Autodesk Inventor part; units mm, degrees
ref_plane "YZ Plane" through (0, 0, 0) normal (1, 0, 0) x (0, 1, 0)
ref_plane "XZ Plane" through (0, 0, 0) normal (0, 1, 0) x (-1, 0, 0)
ref_plane "XY Plane" through (0, 0, 0) normal (0, 0, 1) x (1, 0, 0)
sketch "Sketch1" plane through (0, 0, 0) normal (1, 0, 0) x (0, 1, 0)
  line L0 (0, 0) -> (25.4, 0)
  line L1 (25.4, 0) -> (25.4, -50.8)
  line L2 (25.4, -50.8) -> (0, -50.8)
  line L3 (0, -50.8) -> (0, 0)
  circle A0 centre (12.7, -12.9077) radius 2.75
  circle A1 centre (12.7, -40.4254) radius 2.75
  dimension "d0" = 25.4
  dimension "d1" = 50.8
  dimension "d2" = 5.5
  dimension "d3" = 5.5
extrude "Extrusion1" add sketch "Sketch1" along normal blind 10
sketch "Sketch2" plane through (0, 0, 0) normal (-1, 0, 0) x (0, 0, 1)
  line L0 (-50.8, 0) -> (-50.8, 25.4)
  line L1 (0, 0) -> (-50.8, 0)
  line L2 (0, 25.4) -> (0, 0)
  line L3 (-50.8, 25.4) -> (0, 25.4)
  circle A0 centre (-40.4254, 12.7) radius 2.75
  circle A1 centre (-12.9077, 12.7) radius 2.75
  line L4 (2.3448, 23.6998) -> (5.142, 21.6715)
  line L5 (3.7285, 30.542) -> (1.7002, 27.7448)
  line L6 (20.0524, 42.2345) -> (17.2552, 44.2628)
  line L7 (22.2632, 12.8343) -> (24.2915, 15.6316)
  line L8 (15.4211, 14.2181) -> (18.2183, 12.1898)
  line L9 (0, 25.4) -> (14.9104, 45.963)
  line L10 (14.9104, 45.963) -> (6.8148, 51.8333)
  line L11 (-12.3523, 25.4) -> (6.8148, 51.8333)
  line L12 (0, 25.4) -> (20.563, 10.4896)
  line L13 (20.563, 10.4896) -> (0, 0)
  line L14 (-50.8, 25.4) -> (0, 25.4)
  line L15 (0, 25.4) -> (0, 35.4)
  line L16 (0, 35.4) -> (-50.8, 35.4)
  line L17 (-50.8, 35.4) -> (-50.8, 25.4)
  arc A2 (1.1565, 26.7905) -> (1.5314, 24.4378) centre (3.607, 25.9748) ccw
  arc A3 (1.5161, 27.4909) -> (2.0909, 23.8839) centre (3.607, 25.9748) ccw
  point P0 (-5.1012, 35.4)
  point P1 (1.5314, 24.4378)
  point P2 (1.1565, 26.7905)
extrude "Extrusion2" add sketch "Sketch2" against normal blind 35.4 contours L17 L16 L11 L3 | L2 L12 L4 L8 L13 | L11 L16 L15 L3 | L15 L16 L11 L10 L9 L5 | L9 A3 A2 L12
sketch "Sketch3" plane through (0, 35.4, -5.1012) normal (0, 1, 0) x (1, 0, 0)
  line L0 (0, 0) -> (0, 45.6988)
  line L1 (0, 0) -> (35.4, 0)
  line L2 (35.4, 45.6988) -> (35.4, 0)
  line L3 (0, 45.6988) -> (35.4, 45.6988)
  line L4 (10, 45.6988) -> (10, -5.1012)
  line L5 (10, 45.6988) -> (35.4, 45.6988)
  line L6 (35.4, -5.1012) -> (35.4, 45.6988)
  line L7 (10, -5.1012) -> (35.4, -5.1012)
  line L8 (10, 38.0742) -> (10, 32.5742)
  line L9 (10, 45.6988) -> (10, -5.1012)
  line L10 (10, -5.1012) -> (10, 45.6988)
  line L11 (10, 38.0742) -> (10, 32.5742)
  line L12 (10, 10.5565) -> (10, 5.0565)
  circle A0 centre (22.7, 22.8494) radius 2.75
  point P0 (0, -5.1012)
  dimension "d10" = 5.5
extrude "Extrusion3" cut sketch "Sketch3" against normal blind 35.4 contours A0
sketch "Sketch4" plane through (0, 27.4909, 1.5161) normal (0, -0.587, 0.8096) x (1, 0, 0)
  line L0 (0, -2.5827) -> (35.4, -2.5827)
  line L1 (0, 22.8173) -> (35.4, 22.8173)
  line L2 (0, 22.8173) -> (0, 2.5185)
  line L3 (0, 22.8173) -> (0, -2.5827) construction
  line L4 (7.7, 10.1173) -> (27.7, 10.1173) construction
  line L5 (7.7, 7.5173) -> (27.7, 7.5173)
  line L6 (27.7, 12.7173) -> (7.7, 12.7173)
  arc A0 (7.7, 12.7173) -> (7.7, 7.5173) centre (7.7, 10.1173) ccw
  arc A1 (27.7, 7.5173) -> (27.7, 12.7173) centre (27.7, 10.1173) ccw
  circle A2 centre (7.7, 10.1173) radius 2.6
  circle A3 centre (27.7, 10.1173) radius 2.6
  point P0 (0, -23.1457)
  point P1 (17.7, 10.1173)
  dimension "d13" = 2.6
  dimension "d14" = 20
extrude "Extrusion4" cut sketch "Sketch4" against normal blind 35.4 contours A0 A2 | A3 A1
fillet "Fillet1" radius 10 1 edges at (17.7, 35.4, -5.1012)
fillet "Fillet2" radius 10 4 edges at (0, 48.8982, 10.8626) (35.4, 48.8982, 10.8626) (35.4, 30.4, -50.8) (5, 0, -50.8)
fillet "Fillet3" radius 2 1 edges at (17.7, 10.4896, 20.563)
properties part number "lowerRearBracket"
Here's how the part is built. I have some questions about the finished solid (model axes, mm). A direction names the side the tool comes from. Coordinates: 2 decimals unless noted, no trailing zeros. Order: outer loops, then holes, each group sorted by start corner. A loop starts at its lowest first (then second) coordinate and runs counter-clockwise, first axis right, second up. Notation, with made-up numbers: (84, 52.25) -> (104, 52.25) arc R17 ccw to (104, 61.25) -> close; hole circle Ø4 at (73, 13.25). An arc over 180 degrees is marked (long way). Return JSON: item names as keys, results as strings.
1) If we section it at A-A on z = -35: List the corners of the cut face in (x, y) for me, plus the area to 3 significant figures.
Conclusion:
{"outline": "(0, 0) -> (10, 0) -> (10, 25.4) -> (35.4, 25.4) -> (35.4, 35.4) -> (0, 35.4) -> close", "area": "608 mm²"}
2) If I drill on probe 1 along Z at (x, y) = (7.25, 12.7); probe 2 along Y at (x, z) = (3, -40); probe 3 along X at (y, z) = (22, -38.5), over which ranges is the centre line in solid material (lowest first)?
Conclusion:
{"probe 1": "z = -50.8 to -43.18, -37.68 to -15.66, -10.16 to 17.51", "probe 2": "y = 0 to 9.98, 15.42 to 35.4", "probe 3": "x = 0 to 10"}
3) Thinking about a two-plate mould opening in X: for faces 1 (the cylindrical face through (22.342, 30.47, -30.677)), 2 (the cylindrical face through (32.393, 46.631, 9.132)), 3 (the flat face through (17, 35.4, -30)), which applies, +X half, -X half, draft (parallel to the pull), parting line (faces both ways), or undercut?
Conclusion:
{"face 1": "undercut", "face 2": "+X half", "face 3": "draft"}
4) On a 3-axis mill with a long thin cutter (end or side, diameter ignored), from which of +Z, -Z, +X, -X, +Y, -Y can I reach the whole of each face in a straight line? I mean faces 4 (the flat face through (20, 25.4, -26)), 5 (the cylindrical face through (32.39, 30.33, -47.95)). Say none if no direction works.
Conclusion:
{"face 4": "-Z, +X, -Y", "face 5": "-Z, +X, +Y, -Y"}
5) I'm going to push flat-ended pins straight in: P1, Ø5, axis at x = 32, y = 36, coming from the +Z side; P2, Ø12.5, axis at x = 19.5, y = 9.5, coming from the -Z side; P3, Ø1.5, axis at x = 11, z = -3, coming from the -Y side. Where does each tip first touch, or does it pass through?
Conclusion:
{"P1": "stops at z = 9.5", "P2": "stops at z = 0", "P3": "stops at y = 25.4"}
